Build history of the part. All positions in model axes, mm. Face numbers are marked on the shaded views. A direction names the side the tool comes from. Coordinates: 2 decimals unless noted, no trailing zeros. Order: outer loops, then holes, each group sorted by start corner. A loop starts at its lowest first (then second) coordinate and runs counter-clockwise, first axis right, second up. Notation, with made-up numbers: (33, 10) -> (64, 10) arc R19 cw to (64, 31) -> close; hole circle Ø8 at (46.5, 83.5). An arc over 180 degrees is marked (long way). Write each question's results on one line, items separated by ' | '.
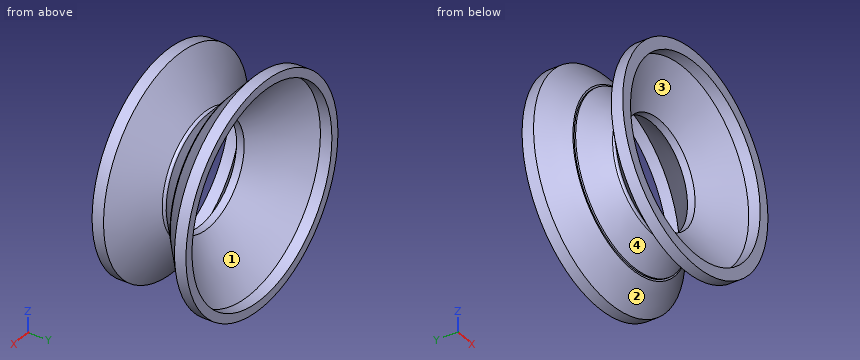
from build123d import *

# Parameters (mm, degrees)
FILLET2_R           = 0.4
SKETCH2_R           = 19.555723827
SKETCH2_R_2         = 18
BOSS_EXTRUDE1_DEPTH = 2
SKETCH3_R           = 18.681949124
SKETCH3_R_2         = 16.681949124
BOSS_EXTRUDE2_DEPTH = 2


with BuildPart() as part:
    # Sketch1 → Revolve1 (revolve)
    with BuildSketch(Plane.XY):
        Polygon((0.662781953, 0), (-4.026073282, 3.934416698), (-4.026073282, 4.195498156), (-4.337218047, 4.195498156), (-8.871246788, 8), (-7.315522961, 8), (1.462781953, 0.634127584), (1.462781953, -0.692820323), (-5.997472085, -5), (-7.997472085, -5), align=None)
    revolve(axis=Axis((10.684477039, 7.609018033, 0), (0, -1, 0)))

    # Fillet2
    fillet2_edges = [part.edges().sort_by_distance(p)[0] for p in [
        (20.706172125, 0, 0),
    ]]
    fillet(fillet2_edges, radius=FILLET2_R)

    # Sketch2 → Boss-Extrude1 (add)
    with BuildSketch(Plane(origin=(0, 8, 0), x_dir=(1, 0, 0), z_dir=(0, 1, 0))):
        with Locations(Location((10.684477039, 0, 0), (0, 0, 180))):
            Circle(SKETCH2_R)
        with Locations(Location((10.684477039, 0, 0), (0, 0, 180))):
            Circle(SKETCH2_R_2, mode=Mode.SUBTRACT)
    extrude(amount=BOSS_EXTRUDE1_DEPTH)

    # Sketch3 → Boss-Extrude2 (add)
    with BuildSketch(Plane.XZ.offset(5)):
        with Locations((10.684477039, 0)):
            Circle(SKETCH3_R)
        with Locations(Location((10.684477039, 0, 0), (0, 0, 180))):
            Circle(SKETCH3_R_2, mode=Mode.SUBTRACT)
    extrude(amount=BOSS_EXTRUDE2_DEPTH)


solid = part.part
Item 1: Pin check, flat tips, straight feed: pin 1 (9 mm diameter, centred on x = 4, z = 5, fed in from -Y); pin 2 (4 mm diameter, centred on x = 13.5, y = -5, fed in from +Z); pin 3 (20 mm diameter, centred on x = 10.68, z = 0, fed in from +Y). Stop position of each tip, or through.
Answer:
pin 1: stops at y = -2.79 | pin 2: stops at z = 18.66 | pin 3: stops at y = 1.29
Item 2: Pull direction Z, two halves, no side cores. Call the marked faces 3 and 4: released by +Z, released by -Z, zero draft, split by the parting line, or undercut.
Answer:
face 3: undercut | face 4: split by the parting line
Item 3: Slice it at A-A, the plane y = -2.75. List the corners of the cut face in (x, z).
Answer:
outline: circle Ø29.57 at (10.68, 0); hole circle Ø25.57 at (10.68, 0)
Item 4: Slice it at B-B, the plane y = 6. List the corners of the cut face in (x, z), and give its area (3 significant figures).
Answer:
outline: circle Ø34.34 at (10.68, 0); hole circle Ø31.23 at (10.68, 0) | area: 160 mm^2
Item 5: Drill centre lines: line 1 (Z direction, x = 11, y = -6); line 2 (Y direction, x = 17.5, z = 17); line 3 (X direction, y = 5.25, z = -7). Where is each one in solid material? Low to high. Write a range as from..to.
Answer:
line 1: z = -18.68..-16.68, 16.68..18.68 | line 2: y = -7..-4.79, 6.96..10 | line 3: x = -4.01..-2.27, 23.64..25.38
Item 6: Tool access for the marked faces 1 and 2: list every direction of +Z, -Z, +X, -X, +Y, -Y with a clear straight run to the whole face (end or side of a thin tool).
Answer:
face 1: +Y | face 2: none
